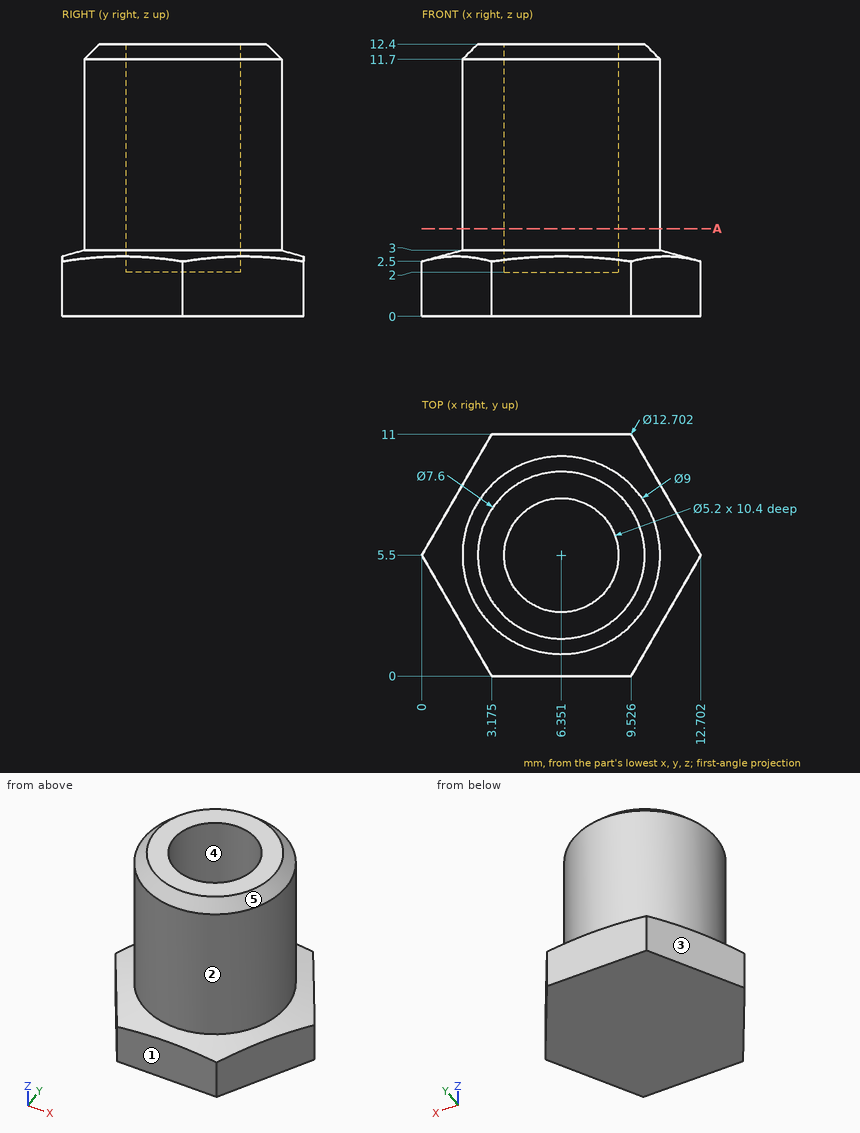
Here's the drawing with two shaded views (mm, measured from the low corner). I have some questions. A direction names the side the tool comes from. Coordinates: 2 decimals unless noted, no trailing zeros. Order: outer loops, then holes, each group sorted by start corner. A loop starts at its lowest first (then second) coordinate and runs counter-clockwise, first axis right, second up.
Item 1: If we section it at A-A, the plane z = 4: List the corners of the cut face in (x, y) for me.
Response values:
outline: circle Ø9 at (6.35, 5.5); hole circle Ø5.2 at (6.35, 5.5)
Item 2: I'm going to push flat-ended pins straight in: pin 1 Ø3 at (x, y) = (2.5, 3) entering from -Z; pin 2 Ø4 at (y, z) = (10, 6) entering from +X; pin 3 Ø4 at (y, z) = (3, 8) entering from +X; pin 4 Ø1 at (x, z) = (6.5, 4) entering from +Y. Where does each tip first touch, or does it pass through?
Response values:
pin 1: stops at z = 0
pin 2: stops at x = 10.09
pin 3: stops at x = 10.82
pin 4: stops at y = 10
Item 3: Which directions (+Z, -Z, +X, -X, +Y, -Y) give clear straight access to the entire face, cutting with the end or side of a thin tool? Please do the marked faces 1 and 2.
Response values:
face 1: +Z, -Z, +X, -X, -Y
face 2: +Z
Item 4: Thinking about a two-plate mould opening in X: for the marked faces 3, 4 and 5, which applies, pulls with the +X half, pulls with the -X half, needs draft (parallel to the pull), parting line crosses it, or undercut?
Response values:
face 3: pulls with the -X half
face 4: undercut
face 5: parting line crosses it
Item 5: I need wall thicknesses on probe 1 along Y at (x, z) = (6.25, 4); probe 2 along Y at (x, z) = (4.5, 5.25) (1 decimal); probe 3 along X at (y, z) = (3.75, 5) (1 decimal). Which ranges of each line are inside material? Lowest first, please.
Response values:
probe 1: y = 1 to 2.9, 8.1 to 10
probe 2: y = 1.4 to 3.7, 7.3 to 9.6
probe 3: x = 2.2 to 4.4, 8.3 to 10.5
